```python
from build123d import *

# Parameters (mm, degrees)
F0_W     = 12
F0_H     = 12
F1_DEPTH = 2
F2_W     = 6.3
F2_H     = 12
F3_DEPTH = 4.15
F4_SIZE  = 1.99999


# Not quite as in the source:
# - a fillet or chamfer is up to 0.001 mm smaller than in the source, because OpenCascade refuses the exact size


with BuildPart() as f1:
    # F0 (on Top) → F1 (new body)
    with BuildSketch(Plane.XY):
        Rectangle(F0_W, F0_H)
    extrude(amount=F1_DEPTH)

    # F2 (on face) → F3 (join)
    with BuildSketch(Plane.XY.offset(2)):
        Rectangle(F2_W, F2_H)
    extrude(amount=F3_DEPTH)

    # F4 (size 2 in the source; OpenCascade refuses exactly that, so slightly less here)
    f4_edges = [f1.edges().sort_by_distance(p)[0] for p in [
        (6, 0, 0),
        (0, -6, 0),
        (-6, 0, 0),
        (0, 6, 0),
    ]]
    chamfer(f4_edges, length=F4_SIZE)


solid = f1.part
```
Read the model definition and answer for the solid it produces. Units are mm, in the model's axes. A direction names the side the tool comes from. Give positions to 0.01 mm unless a question says otherwise; leave off trailing zeros. Write each loop counter-clockwise with the first axis right and the second up, starting at its lowest first coordinate (ties: lowest second). Pieces come first, ordered by that corner, then holes. Notation, with made-up numbers: (63.5, 14) - (113.5, 14) arc R29 cw to (113.5, 51) - close; hole circle Ø9 at (18, -0.75). An arc over 180 degrees is marked (long way). Write item = value, one per line. Start each with the question number.
Item 1: Find the intervals of material crossed by probe 1 along X at (y, z) = (2, 2.5); probe 2 along X at (y, z) = (-2, 0.5); probe 3 along Y at (x, z) = (1, 1.25), in increasing order. Write a range as [from, to].
Item 2: Each of these flat-tipped pins is pushed along its axis until it touches: P1, Ø2, axis at y = 1, z = 4.5, coming from the -X side; P2, Ø1.2, axis at y = 1.5, z = 4.5, coming from the +X side; P3, Ø0.9, axis at x = -4, y = -2, coming from the +Z side. Where does it stop, or does it pass through?
Item 3: A tool of negligible diameter and unlimited length cuts with its end or side. For faces 1 (the flat face through (-3.15, 0, 4)), 2 (the flat face through (0, -5, 1)), 3 (the flat face through (5, 0, 2)), from which of +Z, -Z, +X, -X, +Y, -Y can it reach the whole face along a straight path? Write none if from no direction.
Item 4: Find section C-C (z = 2.5). Give the vertices of the cut face in (x, y), then the cut area to 3 significant figures.
Response:
q1.probe_1 = [-3.15, 3.15]
q1.probe_2 = [-4.5, 4.5]
q1.probe_3 = [-5.25, 5.25]
q2.P1 = -3.15
q2.P2 = 3.15
q2.P3 = 2
q3.face_1 = +Z, -X, +Y, -Y
q3.face_2 = -Z, +X, -X, -Y
q3.face_3 = +Z, +X, +Y, -Y
q4.outline = (-3.15, -6) - (3.15, -6) - (3.15, 6) - (-3.15, 6) - close
q4.area = 75.6 mm²
